CAD build for the part. Positions are in the model's coordinates, mm. A direction names the side the tool comes from. Coordinates: 2 decimals unless noted, no trailing zeros. Loops run counter-clockwise (first coordinate to the right, second up) from the corner with the lowest first, then second, coordinate; pieces in that order, holes last. Notation, with made-up numbers: (-25, 59.25) -> (-4, 59.25) arc R10 ccw to (-4, 78.25) -> close; hole circle Ø8 at (-14, 59.25). An arc over 180 degrees is marked (long way). Return JSON: item names as keys, results as strings. Group by question number.
(1) Flat gauge pins, fed straight in: pin 1 Ø1.5 at (x, z) = (-24.5, -36.5) entering from +Y; pin 2 Ø1.5 at (x, y) = (-30, 1.5) entering from -Z. Where does each tip first touch, or does it go through?
(2) Saw through at A-A on z = 5. Write the cut outline in (x, y) (3 decimals), then the cut area to 3 significant figures.
(3) Tool access for faces 3 (the face through (-41.275, 1.565, 0.169)), 4 (the face through (-31.75, 1.57, 0.23)): list every direction of +Z, -Z, +X, -X, +Y, -Y with a clear straight run to the whole face (end or side of a thin tool).
(4) Saw through at C-C on y = 0.6. Give the number of separate pieces and of enclosed holes in the cut face, then the cut area to 3 significant figures.
(5) Mould opens along Z. For faces 1 (the face through (-9.85, 0, 30.343)), 2 (the face through (-44.107, 1.61, 25.206)) say: pulls with the +Z half, pulls with the -Z half, needs draft (parallel to the pull), parting line crosses it, or undercut.
(6) Probe L1, parallel to Z at x = 0, y = 2.45; L2, parallel to Z at x = 25.5, y = 0.6; L3, parallel to Z at x = -3.5, y = 1.05. List the from-to ranges inside material, lowest first.
(7) Saw through at B-B on x = -4. Write the cut outline in (y, z) (3 decimals), then the cut area to 3 significant figures.
Autodesk Inventor part; units mm, degrees
ref_plane "YZ Plane" through (0, 0, 0) normal (1, 0, 0) x (0, 1, 0)
ref_plane "XZ Plane" through (0, 0, 0) normal (0, 1, 0) x (-1, 0, 0)
ref_plane "XY Plane" through (0, 0, 0) normal (0, 0, 1) x (1, 0, 0)
sketch "Sketch11" plane through (0, 0, 0) normal (0, 1, 0) x (-1, 0, 0)
  circle A0 centre (0, 0) radius 31.75
  circle A1 centre (0, 0) radius 41.275
  dimension "d79" = 63.5
  dimension "d80" = 82.55
extrude "Extrusion10" add sketch "Sketch11" along normal blind 3.175
sketch "Sketch12" plane through (0, 3.175, 0) normal (0, 1, 0) x (1, 0, 0)
  circle A0 centre (0, 0) radius 41.275
  circle A1 centre (0, -41.275) radius 9.5284
  circle A2 centre (35.7452, -20.6375) radius 9.5284
  circle A3 centre (35.7452, 20.6375) radius 9.5284
  circle A4 centre (0, 41.275) radius 9.5284
  circle A5 centre (-35.7452, 20.6375) radius 9.5284
  circle A6 centre (-35.7452, -20.6375) radius 9.5284
  dimension "d85" = 360
extrude "Extrusion11" add sketch "Sketch12" against normal blind 3.175 contours A3 A0 | A0 A3 | A2 A0 | A0 A2 | A4 A0 | A0 A4 | A1 A0 | A0 A1 | A5 A0 | A0 A5 | A6 A0 | A0 A6
sketch "Sketch13" plane through (0, 3.175, 0) normal (0, 1, 0) x (1, 0, 0)
  circle A0 centre (0, -44.45) radius 2.794
  circle A1 centre (38.4948, -22.225) radius 2.794
  circle A2 centre (38.4948, 22.225) radius 2.794
  circle A3 centre (0, 44.45) radius 2.794
  circle A4 centre (-38.4948, 22.225) radius 2.794
  circle A5 centre (-38.4948, -22.225) radius 2.794
  point P0 (0, 0)
  dimension "d89" = 5.588
  dimension "d92" = 360
extrude "Extrusion12" cut sketch "Sketch13" against normal blind 3.175
properties part number "rubber ring"
Geometry results:
{
 "1": {"pin 1": "through", "pin 2": "z = -29.12"},
 "2": {"outline": "(-40.971, 0) -> (-31.354, 0) -> (-31.354, 3.175) -> (-40.971, 3.175) -> close; (31.354, 0) -> (40.971, 0) -> (40.971, 3.175) -> (31.354, 3.175) -> close", "area": "61.1 mm²"},
 "3": {"face 3": "-X, +Y, -Y", "face 4": "+Y, -Y"},
 "4": {"separate pieces": "1", "enclosed holes": "7", "area": "2,940 mm²"},
 "5": {"face 1": "needs draft", "face 2": "undercut"},
 "6": {"L1": "-50.8 to -47.24, -41.66 to -31.75, 31.75 to 41.66, 47.24 to 50.8", "L2": "-32.46 to -18.92, 18.92 to 32.46", "L3": "-50.14 to -31.56, 31.56 to 50.14"},
 "7": {"outline": "(0, -49.923) -> (3.175, -49.923) -> (3.175, -31.497) -> (0, -31.497) -> close; (0, 31.497) -> (3.175, 31.497) -> (3.175, 49.923) -> (0, 49.923) -> close", "area": "117 mm²"}
}
